from build123d import *

# Parameters (mm, degrees)
ESQUISSE1_W             = 93
ESQUISSE1_H             = 72
BOSS_EXTRU_1_DEPTH      = 35.2
ESQUISSE2_R             = 1.75
ENL_V_MAT_EXTRU_1_DEPTH = 123.768236934
ESQUISSE3_R             = 3.5
BOSS_EXTRU_2_DEPTH      = 7


with BuildPart() as part:
    # Esquisse1 → Boss.-Extru.1 (new body)
    with BuildSketch(Plane.XY):
        with Locations((46.5, -36)):
            Rectangle(ESQUISSE1_W, ESQUISSE1_H)
    extrude(amount=BOSS_EXTRU_1_DEPTH)

    # Esquisse2 → Enlèv. mat.-Extru.1 (cut, through all)
    with BuildSketch(Plane(origin=(0, 0, 0), x_dir=(-1, 0, 0), z_dir=(0, 0, -1))):
        with Locations((-89.5, -4)):
            Circle(ESQUISSE2_R)
        with Locations((-3.5, -4)):
            Circle(ESQUISSE2_R)
        with Locations((-89.5, -68)):
            Circle(ESQUISSE2_R)
        with Locations((-3.5, -68)):
            Circle(ESQUISSE2_R)
    extrude(amount=-ENL_V_MAT_EXTRU_1_DEPTH, mode=Mode.SUBTRACT)

    # Esquisse3 → Boss.-Extru.2 (add)
    with BuildSketch(Plane.XY.offset(35.2)):
        with Locations((89.5, -68)):
            Circle(ESQUISSE3_R)
        with Locations(Location((3.5, -68, 0), (0, 0, 180))):
            Circle(ESQUISSE3_R)
        with Locations((89.5, -4)):
            Circle(ESQUISSE3_R)
        with Locations(Location((3.5, -4, 0), (0, 0, 180))):
            Circle(ESQUISSE3_R)
    extrude(amount=BOSS_EXTRU_2_DEPTH)


solid = part.part
Read the model definition and answer for the solid it produces. Units are mm, in the model's axes. A direction names the side the tool comes from. Coordinates: 2 decimals unless noted, no trailing zeros. Write each loop counter-clockwise with the first axis right and the second up, starting at its lowest first coordinate (ties: lowest second). Pieces come first, ordered by that corner, then holes. Notation, with made-up numbers: M -3.5,-11 L 46.5,-11 A21 ccw 46.5,9 Z; hole C 84.5,58.5 d2. An arc over 180 degrees is marked long. Use a Markdown table: item, result.
Q1. Straight lines are drawn through the part: L1, parallel to X at y = -68, z = 22; L2, parallel to Y at x = 3.5, z = 8.5; L3, parallel to Z at x = 46.5, y = -3.5. For each, find the intervals that lie inside material, in ascending order. Write a range as [from, to].
Answer block:
| item | result |
|---|---|
| L1 | x = [0, 1.75], [5.25, 87.75], [91.25, 93] |
| L2 | y = [-72, -69.75], [-66.25, -5.75], [-2.25, 0] |
| L3 | z = [0, 35.2] |
Q2. Each of these flat-tipped pins is pushed along its axis until it touches: pin 1 Ø4 at (x, y) = (89.5, -4.5) entering from -Z; pin 2 Ø3 at (x, y) = (89.5, -68) entering from -Z; pin 3 Ø21.5 at (x, y) = (63.5, -27) entering from +Z. Where does it stop, or does it pass through?
Answer block:
| item | result |
|---|---|
| pin 1 | stops at z = 0 |
| pin 2 | stops at z = 35.2 |
| pin 3 | stops at z = 35.2 |
Q3. Which of the six approach directions +Z, -Z, +X, -X, +Y, -Y give full straight-line access (tool end or side, diameter ignored) to faces 4 (the face through (92.733, -69.341, 38.651)), 5 (the face through (89, -68, 42.2)), 6 (the face through (4, -68, 35.2))?
Answer block:
| item | result |
|---|---|
| face 4 | +Z |
| face 5 | +Z, +X, -X, +Y, -Y |
| face 6 | -Z |
Q4. The part is cut by section B-B, the plane y = -17. Write down the section's boundary in (x, z), then the cut area to 3 significant figures.
Answer block:
| item | result |
|---|---|
| outline | M 0,0 L 93,0 L 93,35.2 L 0,35.2 Z |
| area | 3,270 mm2 |
Q5. The part is cut by section C-C, the plane x = 47.5. Write down the section's boundary in (y, z), then the cut area to 3 significant figures.
Answer block:
| item | result |
|---|---|
| outline | M -72,0 L 0,0 L 0,35.2 L -72,35.2 Z |
| area | 2,530 mm2 |
Q6. The part is cut by section A-A, the plane x = 3.5. Write down the section's boundary in (y, z), then the cut area to 3 significant figures.
Answer block:
| item | result |
|---|---|
| outline | M -72,0 L -69.75,0 L -69.75,35.2 L -66.25,35.2 L -66.25,0 L -5.75,0 L -5.75,35.2 L -2.25,35.2 L -2.25,0 L 0,0 L 0,35.2 L -0.5,35.2 L -0.5,42.2 L -7.5,42.2 L -7.5,35.2 L -64.5,35.2 L -64.5,42.2 L -71.5,42.2 L -71.5,35.2 L -72,35.2 Z |
| area | 2,390 mm2 |
Q7. Determine the mould class of faces 1 (the face through (89.88, -69.71, 17.35)), 2 (the face through (93, -37, 17)), 3 (the face through (46, -72, 17)) for opening direction Y: released by +Y, released by -Y, zero draft, split by the parting line, or undercut.
Answer block:
| item | result |
|---|---|
| face 1 | undercut |
| face 2 | zero draft |
| face 3 | released by -Y |
